```python
from build123d import *

# Parameters (mm, degrees)
SKETCH1_W           = 82
SKETCH1_H           = 60
BOSS_EXTRUDE1_DEPTH = 3
BOSS_EXTRUDE2_DEPTH = 3
SKETCH3_R           = 2.25
SKETCH3_R_2         = 4.75
BOSS_EXTRUDE3_DEPTH = 3
SKETCH4_W           = 7
SKETCH4_H           = 17
CUT_EXTRUDE1_DEPTH  = 3
BOSS_EXTRUDE4_START = -23.5
SKETCH5_W           = 45
SKETCH5_H           = 54.441667663
BOSS_EXTRUDE4_DEPTH = 3
SKETCH6_R           = 2.25
SKETCH6_R_2         = 4.75
CUT_EXTRUDE2_DEPTH  = 3
BOSS_EXTRUDE5_DEPTH = 3
SKETCH8_R           = 1.75
CUT_EXTRUDE3_DEPTH  = 3


with BuildPart() as part:
    # Sketch1 → Boss-Extrude1 (new body)
    with BuildSketch(Plane(origin=(0, 0, 0), x_dir=(1, 0, 0), z_dir=(0, 1, 0))):
        Rectangle(SKETCH1_W, SKETCH1_H)
    extrude(amount=BOSS_EXTRUDE1_DEPTH)

    # Sketch2 → Boss-Extrude2 (add)
    with BuildSketch(Plane.XY.offset(30)):
        Polygon((-41, 0), (-41, 22.5), (-21, 0), align=None)
    boss_extrude2 = extrude(amount=-BOSS_EXTRUDE2_DEPTH)

    # Mirror1: Boss-Extrude2 across plane
    add(boss_extrude2.mirror(Plane.XY))

    # Sketch3 → Boss-Extrude3 (add)
    with BuildSketch(Plane.ZY.offset(41)):
        with BuildLine():
            Line((-30, 0), (30, 0))
            Line((30, 0), (30, 28.236891946))
            ThreePointArc((30, 28.236891946), (0, 58.236891946), (-30, 28.236891946))
            Line((-30, 28.236891946), (-30, 0))
        make_face()
        with Locations((-17.5, 28.236891946)):
            Circle(SKETCH3_R, mode=Mode.SUBTRACT)
        with Locations((17.5, 28.236891946)):
            Circle(SKETCH3_R, mode=Mode.SUBTRACT)
        with Locations((0, 36.236891946)):
            Circle(SKETCH3_R_2, mode=Mode.SUBTRACT)
    extrude(amount=-BOSS_EXTRUDE3_DEPTH)

    # Sketch4 → Cut-Extrude1 (cut)
    with BuildSketch(Plane(origin=(0, 3, 0), x_dir=(1, 0, 0), z_dir=(0, 1, 0))):
        with Locations((-34.5, 0)):
            Rectangle(SKETCH4_W, SKETCH4_H)
    extrude(amount=-CUT_EXTRUDE1_DEPTH, mode=Mode.SUBTRACT)

    # Sketch5 → Boss-Extrude4 (add)
    with BuildSketch(Plane.XY.offset(30).offset(BOSS_EXTRUDE4_START)):
        with Locations((18.5, 27.220833832)):
            Rectangle(SKETCH5_W, SKETCH5_H)
    extrude(amount=-BOSS_EXTRUDE4_DEPTH)

    # Sketch6 → Cut-Extrude2 (cut)
    with BuildSketch(Plane.XY.offset(6.5)):
        with Locations((1, 36.536359397)):
            Circle(SKETCH6_R)
        with Locations((36, 36.536359397)):
            Circle(SKETCH6_R)
        with Locations((18.5, 44.536359397)):
            Circle(SKETCH6_R_2)
    extrude(amount=-CUT_EXTRUDE2_DEPTH, mode=Mode.SUBTRACT)

    # Sketch7 → Boss-Extrude5 (add)
    with BuildSketch(Plane(origin=(41, 0, 0), x_dir=(0, 0, -1), z_dir=(1, 0, 0))):
        Polygon((-21.5, 3), (-6.5, 3), (-6.5, 23), align=None)
        Polygon((-3.5, 3), (11.5, 3), (-3.5, 23), align=None)
    boss_extrude5 = extrude(amount=-BOSS_EXTRUDE5_DEPTH)

    # Mirror2: Boss-Extrude5 across plane
    add(boss_extrude5.mirror(Plane.ZY.offset(-18.5)))

    # Sketch8 → Cut-Extrude3 (cut)
    with BuildSketch(Plane.XZ):
        with Locations(Location((-28.75, 23.25, 0), (0, 0, 270))):
            Circle(SKETCH8_R)
        with Locations(Location((34.25, 23.25, 0), (0, 0, 270))):
            Circle(SKETCH8_R)
        with Locations(Location((34.25, -23.25, 0), (0, 0, 270))):
            Circle(SKETCH8_R)
        with Locations(Location((-28.75, -23.25, 0), (0, 0, 270))):
            Circle(SKETCH8_R)
    extrude(amount=-CUT_EXTRUDE3_DEPTH, mode=Mode.SUBTRACT)


solid = part.part
```
The listing builds one solid part. Answer for the finished solid, in the listing's coordinates (mm). A direction names the side the tool comes from. Round coordinates to 2 decimals unless told otherwise and drop trailing zeros. Loops run counter-clockwise (first coordinate to the right, second up) from the corner with the lowest first, then second, coordinate; pieces in that order, holes last. Notation, with made-up numbers: (-3.5, 33.25) - (22.5, 33.25) arc R22 ccw to (22.5, 43.25) - close; hole circle Ø5 at (-30.75, -34.5). An arc over 180 degrees is marked (long way). Return JSON: item names as keys, results as strings. Group by question number.
1. The part is cut by section C-C on z = 17.5. Determine the outline of the cut face in (x, y), then the cut area to 3 significant figures.
2. Which of the six approach directions +Z, -Z, +X, -X, +Y, -Y give full straight-line access (tool end or side, diameter ignored) to faces 1 (the flat face through (-35, 2, -8.5)), 2 (the flat face through (18, 54.442, 5)), 3 (the flat face through (40, 13, -4)), 4 (the flat face through (18, 29, 3.5)), 5 (the flat face through (1, 3, 0))?
3. The part is cut by section D-D on y = 15.5. Determine the outline of the cut face in (x, z) (3 decimals).
4. Each of these flat-tipped pins is pushed along its axis until it touches: P1, Ø3, axis at x = 22.5, y = 42.5, coming from the -Z side; P2, Ø10, axis at x = -31.5, y = 29.5, coming from the +Z side; P3, Ø3, axis at x = -16.5, z = 13, coming from the -Y side; P4, Ø7, axis at y = 28.24, z = 17.5, coming from the +X side. Where does it stop, or does it pass through?
5. The mould has two halves that part along X. Classify faces 6 (the flat face through (-30.934, 11.175, 28.521)), 7 (the flat face through (-38, 30, 0)), 8 (the cylindrical face through (37.04, 34.54, 5.02)), 9 (the flat face through (-1, 0, 0)): pulls with the +X half, pulls with the -X half, needs draft (parallel to the pull), parting line crosses it, or undercut.
6. Consider probe 1 along X at (y, z) = (6.5, -3); probe 2 along X at (y, z) = (1, 23); probe 3 along Y at (x, z) = (-24, -8). Determine where each line is inside the solid, lowest interval first.
7. The part is cut by section A-A on x = 1. Determine the outline of the cut face in (y, z), then the cut area to 3 significant figures.
8. The part is cut by section B-B on z = 0. Determine the outline of the cut face in (x, y).
Resolved:
{
 "1": {"outline": "(-41, 0) - (41, 0) - (41, 8.33) - (38, 8.33) - (38, 3) - (-1, 3) - (-1, 8.33) - (-4, 8.33) - (-4, 3) - (-38, 3) - (-38, 25.99) - (-41, 25.99) - close; (-41, 30.49) - (-38, 30.49) - (-38, 52.6) - (-41, 52.6) - close", "area": "413 mm²"},
 "2": {"face 1": "+Y, -Y", "face 2": "+Z, -Z, +X, +Y", "face 3": "-Z, +X, +Y", "face 4": "-Z, +Y", "face 5": "+Y"},
 "3": {"outline": "(-41, -30) - (-34.778, -30) - (-34.778, -27) - (-38, -27) - (-38, 27) - (-34.778, 27) - (-34.778, 30) - (-41, 30) - close; (-4, -2.125) - (-1, -2.125) - (-1, 3.5) - (38, 3.5) - (38, -2.125) - (41, -2.125) - (41, 12.125) - (38, 12.125) - (38, 6.5) - (-1, 6.5) - (-1, 12.125) - (-4, 12.125) - close"},
 "4": {"P1": "stops at z = 3.5", "P2": "passes through", "P3": "stops at y = 0", "P4": "stops at x = -38"},
 "5": {"face 6": "pulls with the +X half", "face 7": "undercut", "face 8": "undercut", "face 9": "needs draft"},
 "6": {"probe 1": "x = -41 to -38, -4 to -1, 38 to 41", "probe 2": "x = -41 to -30.48, -27.02 to 32.52, 35.98 to 41", "probe 3": "y = 0 to 3"},
 "7": {"outline": "(0, -30) - (3, -30) - (3, 3.5) - (34.29, 3.5) - (34.29, 6.5) - (3, 6.5) - (3, 30) - (0, 30) - close; (38.79, 3.5) - (54.44, 3.5) - (54.44, 6.5) - (38.79, 6.5) - close", "area": "321 mm²"},
 "8": {"outline": "(-41, 0) - (-38, 0) - (-38, 31.49) - (-41, 31.49) - close; (-41, 40.99) - (-38, 40.99) - (-38, 58.24) - (-41, 58.24) - close; (-31, 0) - (41, 0) - (41, 18.33) - (38, 18.33) - (38, 3) - (-1, 3) - (-1, 18.33) - (-4, 18.33) - (-4, 3) - (-31, 3) - close"}
}
